Could you check a few things on this model? Use its own coordinates, in mm. A direction names the side the tool comes from. Coordinates: 2 decimals unless noted, no trailing zeros. Loops run counter-clockwise (first coordinate to the right, second up) from the corner with the lowest first, then second, coordinate; pieces in that order, holes last. Notation, with made-up numbers: (8, 53.5) -> (63, 53.5) arc R26 ccw to (63, 91.5) -> close; hole circle Ø11 at (-6, 83.25). An arc over 180 degrees is marked (long way). One line per question, with ' | ' between items. Start each with the question number.
(1) I'm going to push flat-ended pins straight in: pin 1 Ø6 at (y, z) = (-6, 14.5) entering from +X; pin 2 Ø2 at (y, z) = (15, 3.5) entering from -X; pin 3 Ø5.5 at (x, z) = (2, 2.5) entering from +Y. Where does each tip first touch, or does it pass through?
(2) Which directions (+Z, -Z, +X, -X, +Y, -Y) give clear straight access to the entire face, cutting with the end or side of a thin tool? Please do faces 4 (the face through (-8.6, 4.91, 2.46)), 5 (the face through (8.57, 4.87, 2.46)), 6 (the face through (-9, 15, 1)), 7 (the face through (-7, 13, 2)).
(3) Suppose I cut it at B-B (y = 11.25). Please give me the cut outline in (x, z).
(4) Suppose I cut it at D-D (z = 14.5). Please give me the cut outline in (x, y) (3 decimals), plus the area to 3 significant figures.
(5) Suppose I cut it at C-C (x = 1.75). Please give me the cut outline in (y, z).
(6) If we mould it in two halves opening along Y, with no side actions, what happens to faces 1 (the face through (9.51, 9, 2)), 2 (the face through (8, 16.798, 2)), 3 (the face through (7.986, 14.644, 1.377))? For each: pulls with the +Y half, pulls with the -Y half, needs draft (parallel to the pull), parting line crosses it, or undercut.
(7) If I drill on line 1 along X through (y, z) = (12.75, 2.5); line 2 along Z through (x, y) = (4.75, 5.75); line 3 along Y through (x, z) = (0.75, 14.75), over which ranges is the centre line in solid material (lowest first)?
(8) Suppose I cut it at A-A (z = 2.5). Give the number of separate pieces and of enclosed holes in the cut face, plus the area to 3 significant figures.
```python
from build123d import *

# Parameters (mm, degrees)
F0_R     = 4.075
F1_DEPTH = 18
F0_W     = 2
F0_H     = 4.459151
F2_DEPTH = 5
F3_DEPTH = 6
F4_R     = 1.15
F5_DEPTH = 25


with BuildPart() as f1:
    # F0 (on Top) → F1 (new body)
    with BuildSketch(Plane.XY):
        with BuildLine():
            ThreePointArc((-6.831683, 1.525812), (-0.767534, -6.957794), (7, 0))
            ThreePointArc((7, 0), (6.957794, 0.767534), (6.831683, 1.525812))
            ThreePointArc((6.831683, 1.525812), (0, 7), (-6.831683, 1.525812))
        make_face()
        Circle(F0_R, mode=Mode.SUBTRACT)
    extrude(amount=F1_DEPTH)

    # F0 (on Top) → F2 (join)
    with BuildSketch(Plane.XY):
        Polygon((-9.510325, 12.338503), (-9.510325, 9), (-7, 9), (-7, 12.338503), (-9, 12.338503), align=None)
        with BuildLine():
            Line((-9.510325, 6.091482), (-7.658741, 3.686961))
            ThreePointArc((-7.658741, 3.686961), (-4.522767, 7.196845), (0, 8.5))
            Line((0, 8.5), (0, 9))
            Line((0, 9), (-7, 9))
            Line((-7, 9), (-9.510325, 9))
            Line((-9.510325, 9), (-9.510325, 6.091482))
        make_face()
        with BuildLine():
            ThreePointArc((-6.831683, 1.525812), (0, 7), (6.831683, 1.525812))
            Line((6.831683, 1.525812), (7.658741, 3.686961))
            ThreePointArc((7.658741, 3.686961), (4.522767, 7.196845), (0, 8.5))
            ThreePointArc((0, 8.5), (-4.522767, 7.196845), (-7.658741, 3.686961))
            Line((-7.658741, 3.686961), (-6.831683, 1.525812))
        make_face()
        with BuildLine():
            ThreePointArc((0, 8.5), (4.522767, 7.196845), (7.658741, 3.686961))
            Line((7.658741, 3.686961), (9.510325, 6.091482))
            Line((9.510325, 6.091482), (9.510325, 9))
            Line((9.510325, 9), (7, 9))
            Line((7, 9), (0, 9))
            Line((0, 9), (0, 8.5))
        make_face()
        Polygon((7, 9), (9.510325, 9), (9.510325, 12.338503), (9, 12.338503), (7, 12.338503), align=None)
        with Locations((-8, 14.568078)):
            Rectangle(F0_W, F0_H)
        with Locations((8, 14.568078)):
            Rectangle(F0_W, F0_H)
    extrude(amount=F2_DEPTH)

    # F0 (on Top) → F3 (join)
    with BuildSketch(Plane.XY):
        with BuildLine():
            ThreePointArc((6.831683, 1.525812), (6.957794, 0.767534), (7, 0))
            ThreePointArc((7, 0), (-0.767534, -6.957794), (-6.831683, 1.525812))
            Line((-6.831683, 1.525812), (-7.658741, 3.686961))
            ThreePointArc((-7.658741, 3.686961), (-1.890859, -8.287017), (8.5, 0))
            ThreePointArc((8.5, 0), (8.287017, 1.890859), (7.658741, 3.686961))
            Line((7.658741, 3.686961), (6.831683, 1.525812))
        make_face()
    extrude(amount=F3_DEPTH)

    # F4 (on face) → F5 (cut)
    with BuildSketch(Plane(origin=(-9, 0, 0), x_dir=(0, -1, 0), z_dir=(-1, 0, 0))):
        with Locations((-14.394956, 2.5)):
            Circle(F4_R)
    extrude(amount=-F5_DEPTH, mode=Mode.SUBTRACT)


solid = f1.part
```
Checks:
1) pin 1: stops at x = 6.32 | pin 2: stops at x = -9 | pin 3: stops at y = 9
2) face 4: +Z, -Z, -X | face 5: +Z, -Z, +X | face 6: +Z, -Z, -X, +Y | face 7: +Z, -Z, +Y
3) outline: (-9.51, 0) -> (-7, 0) -> (-7, 5) -> (-9.51, 5) -> close; (7, 0) -> (9.51, 0) -> (9.51, 5) -> (7, 5) -> close
4) outline: (-6.832, 1.526) arc R7 ccw (long way) to (7, 0) arc R7 ccw to (6.832, 1.526) arc R7 ccw to start; hole circle Ø8.15 at (0, 0) | area: 102 mm^2
5) outline: (-8.32, 0) -> (-3.68, 0) -> (-3.68, 18) -> (-6.78, 18) -> (-6.78, 6) -> (-8.32, 6) -> close; (3.68, 0) -> (9, 0) -> (9, 5) -> (6.78, 5) -> (6.78, 18) -> (3.68, 18) -> close
6) face 1: needs draft | face 2: pulls with the +Y half | face 3: undercut
7) line 1: x = -9 to -7, 7 to 9 | line 2: z = 0 to 5 | line 3: y = -6.96 to -4.01, 4.01 to 6.96
8) separate pieces: 3 | enclosed holes: 1 | area: 244 mm^2
